```python
from build123d import *

# Parameters (mm, degrees)
F1_DEPTH = 25
F2_R     = 2.75
F3_DEPTH = 19.9132636974
F4_R     = 5
F5_DEPTH = 2
F6_DEPTH = 25
F7_W     = 26.5
F7_H     = 18
F8_DEPTH = 61.5532770753


with BuildPart() as f1:
    # F0 (on Top) → F1 (new body)
    with BuildSketch(Plane.XY):
        with BuildLine():
            Line((0, 68.5), (0, 74.5))
            ThreePointArc((0, 74.5), (-35.7787380635, 47.6155391844), (-19.9122636974, 5.7688269843))
            ThreePointArc((-19.9122636974, 5.7688269843), (-10.3655391695, 1.4712619322), (3.09e-08, 0))
            Line((0, 0), (0, 6))
            ThreePointArc((0, 6), (-31.25, 37.25), (0, 68.5))
        make_face()
        with BuildLine():
            ThreePointArc((3.09e-08, 0), (-10.3655391695, 1.4712619322), (-19.9122636974, 5.7688269843))
            Line((-19.9122636974, 5.7688269843), (-19.9122636974, -5.7688269843))
            ThreePointArc((-19.9122636974, -5.7688269843), (-17.5050379591, -4.3693651818), (-15, -3.1536292254))
            ThreePointArc((-15, -3.1536292254), (-7.6639639933, -0.7969321468), (3.09e-08, 0))
        make_face()
        with BuildLine():
            Line((0, -6), (0, 0))
            ThreePointArc((3.09e-08, 0), (-7.6639639933, -0.7969321468), (-15, -3.1536292254))
            Line((-15, -3.1536292254), (-15, -8.0031603575))
            Line((-15, -8.0031603575), (-23.0691324268, -8.0031603575))
            ThreePointArc((-23.0691324268, -8.0031603575), (-27.5276929828, -12.1544103666), (-31.25, -16.9768650673))
            ThreePointArc((-31.25, -16.9768650673), (-37.25, -37.25), (-31.25, -57.5231349327))
            ThreePointArc((-31.25, -57.5231349327), (-25.6133761152, -64.2965795246), (-18.543370794, -69.5564374328))
            Line((-18.543370794, -69.5564374328), (-15, -69.5564374328))
            Line((-15, -69.5564374328), (-15, -71.3463707746))
            ThreePointArc((-15, -71.3463707746), (-7.6639640084, -73.70306785), (0, -74.5))
            Line((0, -74.5), (0, -68.5))
            ThreePointArc((0, -68.5), (-31.25, -37.25), (0, -6))
        make_face()
        with BuildLine():
            ThreePointArc((-18.543370794, -69.5564374328), (-16.7955469217, -70.4986406279), (-15, -71.3463707746))
            Line((-15, -71.3463707746), (-15, -69.5564374328))
            Line((-15, -69.5564374328), (-18.543370794, -69.5564374328))
        make_face()
    extrude(amount=F1_DEPTH)

    # F2 (on face) → F3 (cut, through all)
    with BuildSketch(Plane(origin=(-19.9122636974, 0, 0), x_dir=(0, -1, 0), z_dir=(-1, 0, 0))):
        with Locations((0, 12.5)):
            Circle(F2_R)
    extrude(amount=-F3_DEPTH, mode=Mode.SUBTRACT)

    # F4 (on face) → F5 (cut)
    with BuildSketch(Plane(origin=(-19.9122636974, 0, 0), x_dir=(0, -1, 0), z_dir=(-1, 0, 0))):
        with Locations((0, 12.5)):
            Circle(F4_R)
    extrude(amount=-F5_DEPTH, mode=Mode.SUBTRACT)

    # F0 (on Top) → F6 (join)
    with BuildSketch(Plane.XY):
        with BuildLine():
            ThreePointArc((-31.25, -57.5231349327), (-37.25, -37.25), (-31.25, -16.9768650673))
            Line((-31.25, -16.9768650673), (-31.25, -12.7797988951))
            Line((-31.25, -12.7797988951), (-48.75, -12.7797988951))
            Line((-48.75, -12.7797988951), (-48.75, -64.7797988951))
            Line((-48.75, -64.7797988951), (-31.25, -64.7797988951))
            Line((-31.25, -64.7797988951), (-31.25, -57.5231349327))
        make_face()
        with BuildLine():
            ThreePointArc((-31.25, -16.9768650673), (-27.5276929828, -12.1544103666), (-23.0691324268, -8.0031603575))
            Line((-23.0691324268, -8.0031603575), (-65, -8.0031603575))
            Line((-65, -8.0031603575), (-65, -69.5564374328))
            Line((-65, -69.5564374328), (-18.543370794, -69.5564374328))
            ThreePointArc((-18.543370794, -69.5564374328), (-25.6133761152, -64.2965795246), (-31.25, -57.5231349327))
            Line((-31.25, -57.5231349327), (-31.25, -64.7797988951))
            Line((-31.25, -64.7797988951), (-48.75, -64.7797988951))
            Line((-48.75, -64.7797988951), (-48.75, -12.7797988951))
            Line((-48.75, -12.7797988951), (-31.25, -12.7797988951))
            Line((-31.25, -12.7797988951), (-31.25, -16.9768650673))
        make_face()
        with BuildLine():
            ThreePointArc((-15, -3.1536292254), (-17.5050379591, -4.3693651818), (-19.9122636974, -5.7688269843))
            ThreePointArc((-19.9122636974, -5.7688269843), (-21.5197157184, -6.8449948956), (-23.0691324268, -8.0031603575))
            Line((-23.0691324268, -8.0031603575), (-15, -8.0031603575))
            Line((-15, -8.0031603575), (-15, -3.1536292254))
        make_face()
    extrude(amount=F6_DEPTH)

    # F7 (on face) → F8 (cut, through all)
    with BuildSketch(Plane.XZ.offset(69.5564374328)):
        with Locations((-49.6350233853, 12.2272316366)):
            Rectangle(F7_W, F7_H)
    extrude(amount=-F8_DEPTH, mode=Mode.SUBTRACT)


solid = f1.part
```
Verification items for the finished model (mm, model axes). A direction names the side the tool comes from. Give positions to 0.01 mm unless a question says otherwise; leave off trailing zeros. Order: outer loops, then holes, each group sorted by start corner. A loop starts at its lowest first (then second) coordinate and runs counter-clockwise, first axis right, second up. Notation, with made-up numbers: (8.5, 39) - (54.5, 39) arc R27 ccw to (54.5, 68) - close; hole circle Ø8 at (84, 55). An arc over 180 degrees is marked (long way). Answer as CSV lines item,"result". Start each with the question number.
Item 1: Access from +Z, -Z, +X, -X, +Y, -Y to the whole of each face (thin tool, end or side, straight path). Record for faces 1 (the face through (-34, -8.003, 12)), 2 (the face through (-32, -69.556, 12)), 3 (the face through (-9.082, 2.027, 14.359)), 4 (the face through (-31.242, 36.563, 12.325)), 5 (the face through (-18.926, 4.995, 12.72)).
Item 2: Gauge pin test, flat ends, axial feed: pin 1 (12.5 mm diameter, centred on x = -40.5, z = 16.5, fed in from +Y); pin 2 (8 mm diameter, centred on y = 16, z = 18.5, fed in from -X); pin 3 (8 mm diameter, centred on x = -18, y = 21.5, fed in from +Z); pin 4 (3 mm diameter, centred on y = 6.5, z = 15.5, fed in from -X). Record the tip position at first contact, or that the pin passes through.
Item 3: Section check A-A, the plane z = 5. Record the boundary of the cut face in (x, y).
Item 4: Material ranges on L1, parallel to Z at x = -18, y = 0; L2, parallel to Y at x = -13, z = 9; L3, parallel to Y at x = -19, z = 12.5, recorded low to high.
Item 5: Section check D-D, the plane z = 12.5. Record the boundary of the cut face in (x, y), plus the area to 3 significant figures.
Item 6: Section check B-B, the plane y = -37.25. Record the boundary of the cut face in (x, z).
Item 7: Mould release check, pull along X, two halves, no side actions. Record for faces 6 (the face through (-40, -16, 25)), 7 (the face through (-50, -39, 3.227)), 8 (the face through (-36.385, -39, 12)), 9 (the face through (0, -72, 12)): released by +X, released by -X, zero draft, split by the parting line, or undercut.
Item 8: Section check C-C, the plane x = -45. Record the boundary of the cut face in (y, z), plus the area to 3 significant figures.
Filled in:
1,face 1,"+Z, -Z, -X"
1,face 2,"+Z, -Z, -X, -Y"
1,face 3,"+X, -X"
1,face 4,"+Z, -Z, +X"
1,face 5,"-X"
2,pin 1,"y = 51.9"
2,pin 2,"x = -33.02"
2,pin 3,"through"
2,pin 4,"x = -23.07"
3,outline,"(-65, -69.56) - (-62.89, -69.56) - (-62.89, -8) - (-65, -8) - close; (-36.39, -69.56) - (-18.54, -69.56) arc R37.25 ccw to (0, -74.5) - (0, -68.5) arc R31.25 cw to (0, -6) - (0, 6) arc R31.25 cw to (0, 68.5) - (0, 74.5) arc R37.25 ccw to (-19.91, 5.77) - (-19.91, -5.77) arc R37.25 ccw to (-23.07, -8) - (-36.39, -8) - close"
4,L1,"0 to 7.5, 17.5 to 25"
4,L2,"-72.16 to -65.67, -8.83 to 8.83, 65.67 to 72.16"
4,L3,"-69.56 to -62.06, -12.44 to -5, 5 to 12.44, 62.06 to 69.29"
5,outline,"(-65, -69.56) - (-62.89, -69.56) - (-62.89, -8) - (-65, -8) - close; (-36.39, -69.56) - (-18.54, -69.56) arc R37.25 ccw to (0, -74.5) - (0, -68.5) arc R31.25 cw to (0, -6) - (0, -2.75) - (-17.91, -2.75) - (-17.91, -4.59) arc R37.25 ccw to (-18.64, -5) - (-19.91, -5) - (-19.91, -5.77) arc R37.25 ccw to (-23.07, -8) - (-36.39, -8) - close; (-19.91, 5) - (-17.91, 5) - (-17.91, 2.75) - (0, 2.75) - (0, 6) arc R31.25 cw to (0, 68.5) - (0, 74.5) arc R37.25 ccw to (-19.91, 5.77) - close"
5,area,"1,630 mm^2"
6,outline,"(-65, 0) - (-31.25, 0) - (-31.25, 25) - (-65, 25) - close; hole (-62.89, 3.23) - (-36.39, 3.23) - (-36.39, 21.23) - (-62.89, 21.23) - close"
7,face 6,"zero draft"
7,face 7,"undercut"
7,face 8,"undercut"
7,face 9,"released by +X"
8,outline,"(-69.56, 0) - (-8, 0) - (-8, 3.23) - (-69.56, 3.23) - close; (-69.56, 21.23) - (-8, 21.23) - (-8, 25) - (-69.56, 25) - close"
8,area,"431 mm^2"
